The model under review builds one solid part; all positions refer to its coordinate system, in mm. A direction names the side the tool comes from. Coordinates: 2 decimals unless noted, no trailing zeros. Order: outer loops, then holes, each group sorted by start corner. A loop starts at its lowest first (then second) coordinate and runs counter-clockwise, first axis right, second up. Notation, with made-up numbers: M 2,53.25 L 12,53.25 A17 ccw 12,67.25 Z; hole C 82,-17 d6. An arc over 180 degrees is marked long. Write each question's results on one line, items separated by ' | '.
from build123d import *

# Parameters (mm, degrees)
SKETCH1_R           = 1
BOSS_EXTRUDE1_DEPTH = 4
SKETCH2_W           = 23
SKETCH2_H           = 3
BOSS_EXTRUDE2_DEPTH = 14
CUT_EXTRUDE1_DEPTH  = 116.708871167


with BuildPart() as part:
    # Sketch1 → Boss-Extrude1 (new body)
    with BuildSketch(Plane(origin=(0, 0, 0), x_dir=(1, 0, 0), z_dir=(0, 1, 0))):
        with BuildLine():
            ThreePointArc((-11.5, 10.5), (-19.5, 0), (-11.5, -10.5))
            Line((-11.5, -10.5), (11.5, -10.5))
            ThreePointArc((11.5, -10.5), (61.164895038, -6.360437032), (109.459183673, 5.944011994))
            ThreePointArc((109.459183673, 5.944011994), (110.981730745, 16.501597862), (101.5, 11.615131754))
            ThreePointArc((101.5, 11.615131754), (56.580029181, 4.598574614), (11.5, 10.5))
            Line((11.5, 10.5), (-11.5, 10.5))
        make_face()
        with Locations(Location((-14.5, 0, 0), (0, 0, 270))):
            Circle(SKETCH1_R, mode=Mode.SUBTRACT)
        Polygon((11.5, -6.5), (-11.5, -6.5), (-11.5, -3), (-12.5, -3), (-12.5, 3), (-11.5, 3), (-11.5, 6.5), (11.5, 6.5), align=None, mode=Mode.SUBTRACT)
        with Locations(Location((14.5, 0, 0), (0, 0, 270))):
            Circle(SKETCH1_R, mode=Mode.SUBTRACT)
        with BuildLine():
            Line((17.5, -6.5), (17.5, 5.5))
            ThreePointArc((17.5, 5.5), (47.290216061, 0.482498836), (77.5, 0.517787187))
            ThreePointArc((77.5, 0.517787187), (47.704508509, -4.739593528), (17.5, -6.5))
        make_face(mode=Mode.SUBTRACT)
    extrude(amount=BOSS_EXTRUDE1_DEPTH)

    # Sketch2 → Boss-Extrude2 (add)
    with BuildSketch(Plane(origin=(0, 4, 0), x_dir=(1, 0, 0), z_dir=(0, 1, 0))):
        with Locations((0, -8)):
            Rectangle(SKETCH2_W, SKETCH2_H)
        with Locations((0, 8)):
            Rectangle(SKETCH2_W, SKETCH2_H)
    extrude(amount=BOSS_EXTRUDE2_DEPTH)

    # Sketch3 → Cut-Extrude1 (cut, through all)
    with BuildSketch(Plane(origin=(0, 4, 0), x_dir=(1, 0, 0), z_dir=(0, 1, 0))):
        with BuildLine():
            Line((102.276706609, 14.567623271), (105.378679656, 13.736452098))
            Line((105.378679656, 13.736452098), (104.547508484, 16.838425145))
            ThreePointArc((104.547508484, 16.838425145), (103.257359313, 15.857772441), (102.276706609, 14.567623271))
        make_face()
        with BuildLine():
            ThreePointArc((110.54725901, 16.783711107), (109.052914271, 17.410686712), (107.445285962, 17.61488228))
            Line((107.445285962, 17.61488228), (108.276457135, 14.512909233))
            Line((108.276457135, 14.512909233), (110.54725901, 16.783711107))
        make_face()
        with BuildLine():
            ThreePointArc((113.499750526, 11.560417717), (113.295554958, 13.168046025), (112.668579353, 14.662390764))
            Line((112.668579353, 14.662390764), (110.397777479, 12.391588889))
            Line((110.397777479, 12.391588889), (113.499750526, 11.560417717))
        make_face()
        with BuildLine():
            ThreePointArc((110.452491516, 6.391838363), (111.742640687, 7.372491067), (112.723293391, 8.662640238))
            Line((112.723293391, 8.662640238), (109.621320344, 9.493811411))
            Line((109.621320344, 9.493811411), (110.452491516, 6.391838363))
        make_face()
    extrude(amount=-CUT_EXTRUDE1_DEPTH, mode=Mode.SUBTRACT)


solid = part.part
1) Take a section at C-C on z = 5. State the section outline as (x, y) points.
Solutions:
outline: M -18.28,0 L -11.5,0 L -11.5,4 L -18.28,4 Z; M 11.5,0 L 17.5,0 L 17.5,4 L 11.5,4 Z; M 45.39,0 L 68.68,0 L 68.68,4 L 45.39,4 Z
2) For faces 1 (the flat face through (0, 2, -10.5)), 2 (the flat face through (0, 11, -9.5)), 3 (the flat face through (11.5, 2, 0)), 4 (the flat face through (11.5, 11, 8)), 5 (the flat face through (0, 11, 9.5)), list the 3-axis set-ups (+Z, -Z, +X, -X, +Y, -Y) from which the entire face can be reached by the end or side of a thin tool; tool diameter is ignored.
Solutions:
face 1: -Z, -X, +Y, -Y | face 2: -Z, +X, -X, +Y | face 3: +Y, -Y | face 4: +Z, -Z, +X, +Y | face 5: +Z, +X, -X, +Y
3) Take a section at A-A on y = 8. State the section outline as (x, z) points, plus the area to 3 significant figures.
Solutions:
outline: M -11.5,-9.5 L 11.5,-9.5 L 11.5,-6.5 L -11.5,-6.5 Z; M -11.5,6.5 L 11.5,6.5 L 11.5,9.5 L -11.5,9.5 Z | area: 138 mm2
4) For pin 1 (10 mm diameter, centred on x = 40, z = -4.5, fed in from +Y); pin 2 (1.1 mm diameter, centred on x = -12, y = 2.5, fed in from -Z); pin 3 (10 mm diameter, centred on y = 12.5, z = 1, fed in from +X); pin 4 (2.5 mm diameter, centred on y = 8.5, z = 8, fed in from +X), all flat-tipped, find the tip position at first contact; note any pin that passes through.
Solutions:
pin 1: y = 4 | pin 2: z = -10.5 | pin 3: through | pin 4: x = 11.5
5) To check wall thickness, follow line 1 along Z through (x, y) = (-1.5, 7.5); line 2 along Y through (x, z) = (10, 9.75); line 3 along Z through (x, y) = (69.5, 1.75). State the ranges of each line that lie inside material, in increasing order.
Solutions:
line 1: -9.5 to -6.5, 6.5 to 9.5 | line 2: 0 to 4 | line 3: -5.28 to -0.01, 1.25 to 4.84
6) The part is to be moulded in two halves that separate along X. For faces 6 (the flat face through (111.194, 2.028, -9.072)), 7 (the flat face through (-11.5, 11, -8)), 8 (the cylindrical face through (113.29, 1.97, -10.04)), 9 (the flat face through (103.806, 2.028, -14.158)), say which applies: pulls with the +X half, pulls with the -X half, needs draft (parallel to the pull), parting line crosses it, or undercut.
Solutions:
face 6: undercut | face 7: pulls with the -X half | face 8: pulls with the +X half | face 9: undercut
7) Take a section at B-B on x = 71. State the section outline as (y, z) points.
Solutions:
outline: M 0,-5.43 L 4,-5.43 L 4,-0.08 L 0,-0.08 Z; M 0,0.94 L 4,0.94 L 4,4.54 L 0,4.54 Z
